Read the model definition and answer for the solid it produces. Units are mm, in the model's axes. Face numbers are marked on the shaded views. A direction names the side the tool comes from. Give positions to 0.01 mm unless a question says otherwise; leave off trailing zeros. Write each loop counter-clockwise with the first axis right and the second up, starting at its lowest first coordinate (ties: lowest second). Pieces come first, ordered by that corner, then holes. Notation, with made-up numbers: (24, -5) -> (43, -5) arc R24 cw to (43, 32) -> close; hole circle Ø7 at (84, 88.25). An arc over 180 degrees is marked (long way). Use a Markdown table: item, result.
from build123d import *

# Parameters (mm, degrees)
SKETCH1_W           = 55.75
SKETCH1_H           = 25
SKETCH1_R           = 4
SKETCH1_R_2         = 1.5
SKETCH1_R_3         = 1
BOSS_EXTRUDE1_DEPTH = 2
SKETCH2_W           = 2
SKETCH2_H           = 25
BOSS_EXTRUDE2_DEPTH = 62.5
FILLET1_R           = 3
CUT_EXTRUDE1_DEPTH  = 56
SKETCH4_R           = 4
SKETCH4_R_2         = 1.5
SKETCH4_R_3         = 1
CUT_EXTRUDE2_DEPTH  = 56


with BuildPart() as part:
    # Sketch1 → Boss-Extrude1 (new body)
    with BuildSketch(Plane(origin=(0, 0, 0), x_dir=(1, 0, 0), z_dir=(0, 1, 0))):
        with Locations((27.875, 12.5)):
            Rectangle(SKETCH1_W, SKETCH1_H)
        with Locations(Location((27.875, 12.5, 0), (0, 0, 270))):
            Circle(SKETCH1_R, mode=Mode.SUBTRACT)
        with Locations(Location((27.875, 19.4, 0), (0, 0, 270))):
            Circle(SKETCH1_R_2, mode=Mode.SUBTRACT)
        with Locations(Location((34.775, 12.5, 0), (0, 0, 270))):
            Circle(SKETCH1_R_2, mode=Mode.SUBTRACT)
        with Locations(Location((27.875, 5.6, 0), (0, 0, 270))):
            Circle(SKETCH1_R_2, mode=Mode.SUBTRACT)
        with Locations(Location((20.975, 12.5, 0), (0, 0, 270))):
            Circle(SKETCH1_R_2, mode=Mode.SUBTRACT)
        with Locations(Location((32.683326112, 17.308326112, 0), (0, 0, 270))):
            Circle(SKETCH1_R_3, mode=Mode.SUBTRACT)
        with Locations(Location((32.683326112, 7.691673888, 0), (0, 0, 270))):
            Circle(SKETCH1_R_3, mode=Mode.SUBTRACT)
        with Locations(Location((23.066673888, 7.691673888, 0), (0, 0, 270))):
            Circle(SKETCH1_R_3, mode=Mode.SUBTRACT)
        with Locations(Location((23.066673888, 17.308326112, 0), (0, 0, 270))):
            Circle(SKETCH1_R_3, mode=Mode.SUBTRACT)
        with Locations(Location((46.375, 12.5, 0), (0, 0, 270))):
            Circle(SKETCH1_R_2, mode=Mode.SUBTRACT)
        with Locations(Location((9.375, 12.5, 0), (0, 0, 90))):
            Circle(SKETCH1_R_2, mode=Mode.SUBTRACT)
    extrude(amount=BOSS_EXTRUDE1_DEPTH)

    # Sketch2 → Boss-Extrude2 (add)
    with BuildSketch(Plane(origin=(0, 2, 0), x_dir=(1, 0, 0), z_dir=(0, 1, 0))):
        with Locations((1, 12.5)):
            Rectangle(SKETCH2_W, SKETCH2_H)
        with Locations((54.75, 12.5)):
            Rectangle(SKETCH2_W, SKETCH2_H)
    extrude(amount=BOSS_EXTRUDE2_DEPTH)

    # Fillet1
    fillet1_edges = [part.edges().sort_by_distance(p)[0] for p in [
        (55.75, 0, -12.5),
        (0, 0, -12.5),
    ]]
    fillet(fillet1_edges, radius=FILLET1_R)

    # Sketch3 → Cut-Extrude1 (cut)
    with BuildSketch(Plane(origin=(55.75, 0, 0), x_dir=(0, 0, -1), z_dir=(1, 0, 0))):
        with BuildLine():
            Line((12.5, 64.5), (0, 64.5))
            Line((0, 64.5), (0, 52))
            ThreePointArc((0, 52), (3.661165235, 60.838834765), (12.5, 64.5))
        make_face()
        with BuildLine():
            Line((25, 64.5), (12.5, 64.5))
            ThreePointArc((12.5, 64.5), (21.338834765, 60.838834765), (25, 52))
            Line((25, 52), (25, 64.5))
        make_face()
    extrude(amount=-CUT_EXTRUDE1_DEPTH, mode=Mode.SUBTRACT)

    # Sketch4 → Cut-Extrude2 (cut)
    with BuildSketch(Plane(origin=(55.75, 0, 0), x_dir=(0, 0, -1), z_dir=(1, 0, 0))):
        with Locations((12.5, 52)):
            Circle(SKETCH4_R)
        with Locations((5.6, 52)):
            Circle(SKETCH4_R_2)
        with Locations((12.5, 58.9)):
            Circle(SKETCH4_R_2)
        with Locations((19.4, 52)):
            Circle(SKETCH4_R_2)
        with Locations((12.5, 45.1)):
            Circle(SKETCH4_R_2)
        with Locations((7.691673888, 47.191673888)):
            Circle(SKETCH4_R_3)
        with Locations((12.5, 33.7)):
            Circle(SKETCH4_R_2)
        with Locations((12.5, 16.7)):
            Circle(SKETCH4_R_2)
        with Locations((7.691673888, 56.808326112)):
            Circle(SKETCH4_R_3)
        with Locations((17.308326112, 56.808326112)):
            Circle(SKETCH4_R_3)
        with Locations((17.308326112, 47.191673888)):
            Circle(SKETCH4_R_3)
    extrude(amount=-CUT_EXTRUDE2_DEPTH, mode=Mode.SUBTRACT)


solid = part.part
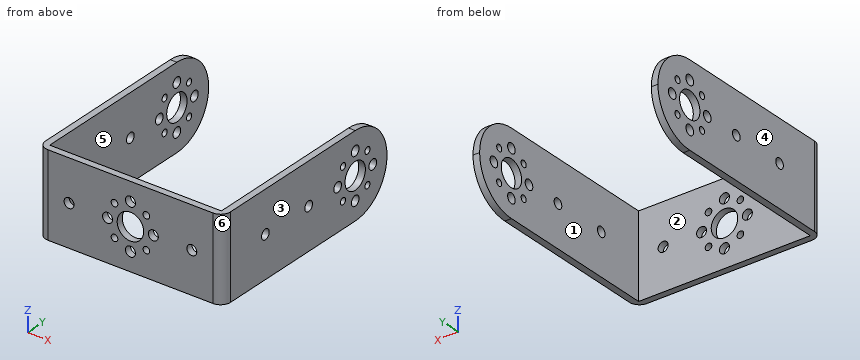
Item 1: A cutting plane is placed at A-A (y = 16.7). Give the vertices of the cut face in (x, z).
Return value:
| item | result |
|---|---|
| outline | (0, -25) -> (2, -25) -> (2, -14) -> (0, -14) -> close; (0, -11) -> (2, -11) -> (2, 0) -> (0, 0) -> close; (53.75, -25) -> (55.75, -25) -> (55.75, -14) -> (53.75, -14) -> close; (53.75, -11) -> (55.75, -11) -> (55.75, 0) -> (53.75, 0) -> close |
Item 2: Each of these flat-tipped pins is pushed along its axis until it touches: P1, Ø2, axis at x = 18, z = -7.5, coming from the +Y side; P2, Ø5, axis at y = 58.9, z = -12.5, coming from the -X side; P3, Ø1.8, axis at y = 33.7, z = -12.5, coming from the +X side. Where does it stop, or does it pass through?
Return value:
| item | result |
|---|---|
| P1 | y = 2 |
| P2 | x = 0 |
| P3 | through |
Item 3: A tool of negligible diameter and unlimited length cuts with its end or side. For the marked faces 5 and 6, from which of +Z, -Z, +X, -X, +Y, -Y can it reach the whole face along a straight path? Write none if from no direction.
Return value:
| item | result |
|---|---|
| face 5 | +Z, -Z, +Y |
| face 6 | +Z, -Z, +X, -Y |
Item 4: For a pull along X with two mould halves and no side action, classify the marked faces 1, 2, 3 and 4 as +X half, -X half, draft (parallel to the pull), parting line (faces both ways), or undercut.
Return value:
| item | result |
|---|---|
| face 1 | undercut |
| face 2 | undercut |
| face 3 | +X half |
| face 4 | -X half |
Item 5: A cutting plane is placed at D-D (y = 58.9). Give the vertices of the cut face in (x, z).
Return value:
| item | result |
|---|---|
| outline | (0, -22.92) -> (2, -22.92) -> (2, -14) -> (0, -14) -> close; (0, -11) -> (2, -11) -> (2, -2.08) -> (0, -2.08) -> close; (53.75, -22.92) -> (55.75, -22.92) -> (55.75, -14) -> (53.75, -14) -> close; (53.75, -11) -> (55.75, -11) -> (55.75, -2.08) -> (53.75, -2.08) -> close |
Item 6: Straight lines are drawn through the part: line 1 along X through (y, z) = (24, -21); line 2 along X through (y, z) = (0.5, -12.5) (3 decimals); line 3 along Y through (x, z) = (37, -4). For each, find the intervals that lie inside material, in ascending order. Write a range as [from, to].
Return value:
| item | result |
|---|---|
| line 1 | [0, 2], [53.75, 55.75] |
| line 2 | [1.342, 7.875], [10.875, 19.475], [22.475, 23.875], [31.875, 33.275], [36.275, 44.875], [47.875, 54.408] |
| line 3 | [0, 2] |
Item 7: A cutting plane is placed at C-C (x = 12.5). Give the vertices of the cut face in (y, z), then the cut area to 3 significant figures.
Return value:
| item | result |
|---|---|
| outline | (0, -25) -> (2, -25) -> (2, 0) -> (0, 0) -> close |
| area | 50.0 mm^2 |
Item 8: A cutting plane is placed at B-B (z = -5.6). Give the vertices of the cut face in (x, y) (3 decimals), then the cut area to 3 significant figures.
Return value:
| item | result |
|---|---|
| outline | (0, 3) arc R3 ccw to (3, 0) -> (26.375, 0) -> (26.375, 2) -> (2, 2) -> (2, 50.5) -> (0, 50.5) -> close; (0, 53.5) -> (2, 53.5) -> (2, 62.423) -> (0, 62.423) -> close; (29.375, 0) -> (52.75, 0) arc R3 ccw to (55.75, 3) -> (55.75, 50.5) -> (53.75, 50.5) -> (53.75, 2) -> (29.375, 2) -> close; (53.75, 53.5) -> (55.75, 53.5) -> (55.75, 62.423) -> (53.75, 62.423) -> close |
| area | 331 mm^2 |
